Here's the drawing with two shaded views (mm, measured from the low corner). I have some questions. A direction names the side the tool comes from. Round coordinates to 2 decimals unless told otherwise and drop trailing zeros. Loops run counter-clockwise (first coordinate to the right, second up) from the corner with the lowest first, then second, coordinate; pieces in that order, holes last. Notation, with made-up numbers: (23.5, 65.5) - (61.5, 65.5) arc R32 ccw to (61.5, 95.5) - close; hole circle Ø7 at (56.5, 59.5). An arc over 180 degrees is marked (long way). Answer as CSV lines item,"result".
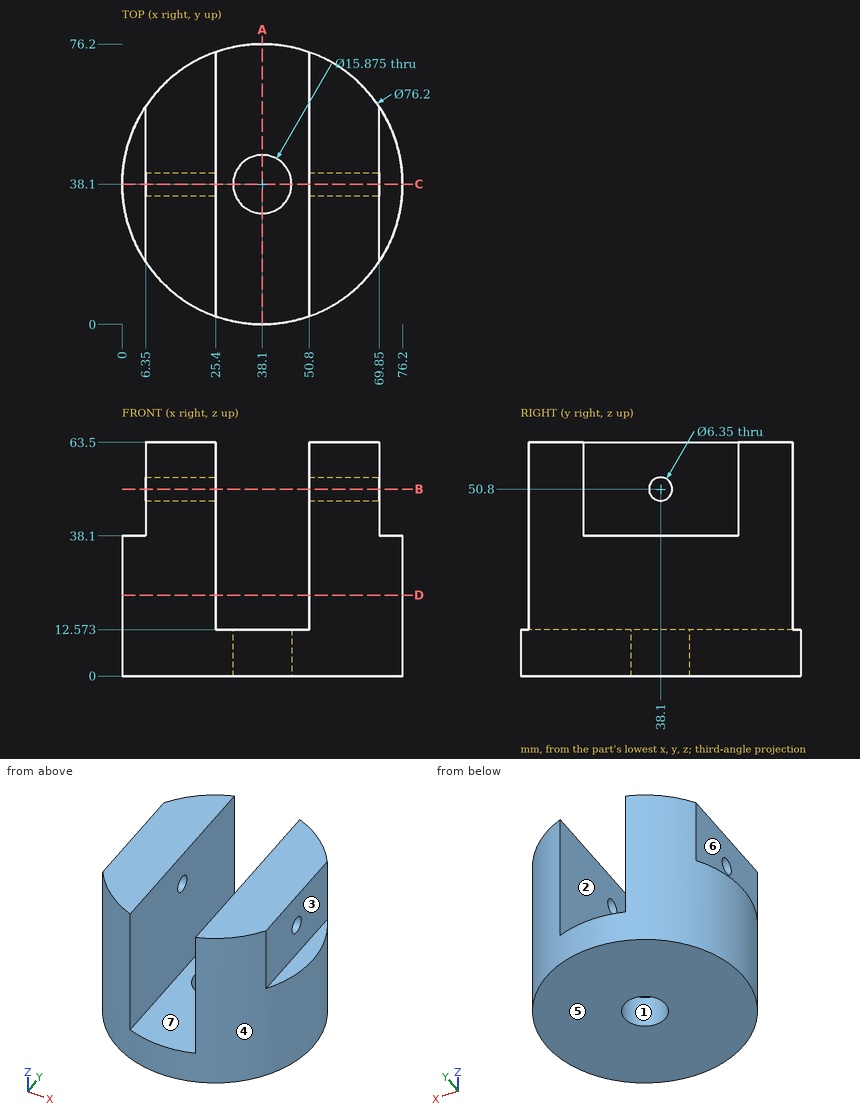
Q1. Imagine slicing it at D-D (z = 22). Write out the boundary of the cut face in (x, y).
Checks:
outline,"(25.4, 2.18) - (25.4, 74.02) arc R38.1 ccw to start; (50.8, 2.18) arc R38.1 ccw to (50.8, 74.02) - close"
Q2. If I drill on line 1 along X through (y, z) = (38, 7); line 2 along X through (y, z) = (52, 54.5), over which ranges is the centre line in solid material (lowest first)? Write a range as [from, to].
Checks:
line 1,"[0, 30.16], [46.04, 76.2]"
line 2,"[6.35, 25.4], [50.8, 69.85]"
Q3. We'd pull the mould along X, two halves only. Please class the marked faces 4, 5, 6 and 7: pulls with the +X half, pulls with the -X half, needs draft (parallel to the pull), parting line crosses it, or undercut.
Checks:
face 4,"parting line crosses it"
face 5,"needs draft"
face 6,"pulls with the -X half"
face 7,"undercut"
Q4. I'm going to push flat-ended pins straight in: pin 1 Ø12 at (y, z) = (64.5, 38.5) entering from +X; pin 2 Ø8 at (y, z) = (67, 37.5) entering from -X; pin 3 Ø1.5 at (x, y) = (25.5, 32) entering from -Z; pin 4 Ø3 at (y, z) = (61.5, 50.5) entering from +X. Where does each tip first touch, or does it pass through?
Checks:
pin 1,"x = 70.27"
pin 2,"x = 9.26"
pin 3,"z = 0"
pin 4,"x = 69.28"
Q5. Imagine slicing it at A-A (x = 38.1). Write out the boundary of the cut face in (y, z).
Checks:
outline,"(0, 0) - (30.16, 0) - (30.16, 12.57) - (0, 12.57) - close; (46.04, 0) - (76.2, 0) - (76.2, 12.57) - (46.04, 12.57) - close"
Q6. On a 3-axis mill with a long thin cutter (end or side, diameter ignored), from which of +Z, -Z, +X, -X, +Y, -Y can I reach the whole of each face in a straight line? I mean the marked faces 1, 2 and 3. Say none if no direction works.
Checks:
face 1,"+Z, -Z"
face 2,"+Z, +Y, -Y"
face 3,"+Z, +X, +Y, -Y"
Q7. Imagine slicing it at B-B (z = 50.8). Write out the boundary of the cut face in (x, y) (3 decimals).
Checks:
outline,"(6.35, 17.039) arc R38.1 ccw to (25.4, 2.179) - (25.4, 34.925) - (6.35, 34.925) - close; (6.35, 41.275) - (25.4, 41.275) - (25.4, 74.021) arc R38.1 ccw to (6.35, 59.161) - close; (50.8, 2.179) arc R38.1 ccw to (69.85, 17.039) - (69.85, 34.925) - (50.8, 34.925) - close; (50.8, 41.275) - (69.85, 41.275) - (69.85, 59.161) arc R38.1 ccw to (50.8, 74.021) - close"
Q8. Imagine slicing it at C-C (y = 38.1). Count the separate pieces of the cut face and the enclosed holes in it, then the cut area to 3 significant figures.
Checks:
separate pieces,"4"
enclosed holes,"0"
area,"2,780 mm²"
